Geometry: final body of the model. Coordinates: model frame, mm. A direction names the side the tool comes from. Give positions to 0.01 mm unless a question says otherwise; leave off trailing zeros. Order: outer loops, then holes, each group sorted by start corner. A loop starts at its lowest first (then second) coordinate and runs counter-clockwise, first axis right, second up. Notation, with made-up numbers: (-31, 22.25) - (-6, 22.25) arc R33 cw to (-6, 54.25) - close; hole circle Ø10 at (-8, 10). An arc over 180 degrees is marked (long way). Put each result on its own line as item: value. Start each with the question number.
1. First-contact query: P1, Ø12, axis at x = 9, y = -21, coming from the -Z side. Flat tip, straight axial feed; report the tip coordinate or a pass-through.
2. Section A-A on y = 0. Return the cut outline in (x, z), plus the area to 3 significant figures.
3. Set-up query: faces 1 (the flat face through (-37, -1, -291)), 2 (the cylindrical face through (-5.5, -24.9, -4.9)). Return all of +Z, -Z, +X, -X, +Y, -Y with unobstructed straight access to the full face (end or side cutting, diameter ignored); none if empty.
4. Ray query, line 1 along Y through (x, z) = (0, -8); line 2 along Y through (x, z) = (19.5, -534). Return the intervals inside material, ascending. Write a range as from..to.
5. Section C-C on z = -464.5. Return the cut outline in (x, y), plus the area to 3 significant figures.
6. Mould query, pull axis Y, two halves, no side actions, for faces 3 (the flat face through (-18.3, 18.3, 0)), 4 (the flat face through (37, 1, -291)), 5 (the flat face through (1, 40, -286)). Classes: pulls with the +Y half, pulls with the -Y half, needs draft (parallel to the pull), parting line crosses it, or undercut.
from build123d import *

# Parameters (mm, degrees)
F1_DEPTH = 580
F0_R     = 25.5
F2_DEPTH = 10


with BuildPart() as f1:
    # F0 (on Top) → F1 (new body)
    with BuildSketch(Plane.XY):
        with BuildLine():
            ThreePointArc((40, 36), (38.828427, 38.828427), (36, 40))
            Line((36, 40), (-36, 40))
            ThreePointArc((-36, 40), (-38.828427, 38.828427), (-40, 36))
            Line((-40, 36), (-40, -36))
            ThreePointArc((-40, -36), (-38.828427, -38.828427), (-36, -40))
            Line((-36, -40), (36, -40))
            ThreePointArc((36, -40), (38.828427, -38.828427), (40, -36))
            Line((40, -36), (40, 36))
        make_face()
        with BuildLine():
            ThreePointArc((-37, 36), (-36.707107, 36.707107), (-36, 37))
            Line((-36, 37), (36, 37))
            ThreePointArc((36, 37), (36.707107, 36.707107), (37, 36))
            Line((37, 36), (37, -36))
            ThreePointArc((37, -36), (36.707107, -36.707107), (36, -37))
            Line((36, -37), (-36, -37))
            ThreePointArc((-36, -37), (-36.707107, -36.707107), (-37, -36))
            Line((-37, -36), (-37, 36))
        make_face(mode=Mode.SUBTRACT)
    extrude(amount=-F1_DEPTH)

    # F0 (on Top) → F2 (join)
    with BuildSketch(Plane.XY):
        with BuildLine():
            Line((36, 37), (-36, 37))
            ThreePointArc((-36, 37), (-36.707107, 36.707107), (-37, 36))
            Line((-37, 36), (-37, -36))
            ThreePointArc((-37, -36), (-36.707107, -36.707107), (-36, -37))
            Line((-36, -37), (36, -37))
            ThreePointArc((36, -37), (36.707107, -36.707107), (37, -36))
            Line((37, -36), (37, 36))
            ThreePointArc((37, 36), (36.707107, 36.707107), (36, 37))
        make_face()
        Circle(F0_R, mode=Mode.SUBTRACT)
    extrude(amount=-F2_DEPTH)


solid = f1.part
Resolved:
1. P1: z = -10
2. outline: (-40, -580) - (-37, -580) - (-37, -10) - (-25.5, -10) - (-25.5, 0) - (-40, 0) - close; (25.5, -10) - (37, -10) - (37, -580) - (40, -580) - (40, 0) - (25.5, 0) - close
2. area: 3,710 mm^2
3. face 1: -Z
3. face 2: +Z, -Z
4. line 1: -40..-25.5, 25.5..40
4. line 2: -40..-37, 37..40
5. outline: (-40, -36) arc R4 ccw to (-36, -40) - (36, -40) arc R4 ccw to (40, -36) - (40, 36) arc R4 ccw to (36, 40) - (-36, 40) arc R4 ccw to (-40, 36) - close; hole (-37, -36) arc R1 ccw to (-36, -37) - (36, -37) arc R1 ccw to (37, -36) - (37, 36) arc R1 ccw to (36, 37) - (-36, 37) arc R1 ccw to (-37, 36) - close
5. area: 911 mm^2
6. face 3: needs draft
6. face 4: undercut
6. face 5: pulls with the +Y half
